Here's how the part is built. I have some questions about the finished solid (model axes, mm). Round coordinates to 2 decimals unless told otherwise and drop trailing zeros. Loops run counter-clockwise (first coordinate to the right, second up) from the corner with the lowest first, then second, coordinate; pieces in that order, holes last. Notation, with made-up numbers: M -7.75,20 L 13.25,20 A16 cw 13.25,48 Z; hole C -13.5,54 d8. An arc over 180 degrees is marked long. One line per question, with ' | ' between items. Start each with the question number.
```python
from build123d import *

# Parameters (mm, degrees)
SKETCH1_R           = 31
BOSS_EXTRUDE1_DEPTH = 2
SKETCH2_R           = 6
CUT_EXTRUDE1_DEPTH  = 2
SKETCH3_W           = 16
SKETCH3_H           = 62
BOSS_EXTRUDE2_DEPTH = 2
CUT_EXTRUDE2_REACH  = 71.347
SKETCH11_R          = 1


with BuildPart() as part:
    # Sketch1 → Boss-Extrude1 (new body)
    with BuildSketch(Plane(origin=(0, 0, 0), x_dir=(1, 0, 0), z_dir=(0, 1, 0))):
        with Locations(Location((0, 0, 0), (0, 0, 270))):
            Circle(SKETCH1_R)
    extrude(amount=BOSS_EXTRUDE1_DEPTH)

    # Sketch2 → Cut-Extrude1 (cut)
    with BuildSketch(Plane(origin=(0, 2, 0), x_dir=(1, 0, 0), z_dir=(0, 1, 0))):
        with Locations(Location((0, 0, 0), (0, 0, 270))):
            Circle(SKETCH2_R)
    extrude(amount=-CUT_EXTRUDE1_DEPTH, mode=Mode.SUBTRACT)

    # Sketch3 → Boss-Extrude2 (add)
    with BuildSketch(Plane(origin=(0, 2, 0), x_dir=(1, 0, 0), z_dir=(0, 1, 0))):
        with Locations((-23, 31)):
            Rectangle(SKETCH3_W, SKETCH3_H)
    extrude(amount=-BOSS_EXTRUDE2_DEPTH)

    # Sketch11 → Cut-Extrude2 (cut, up to next)
    with BuildSketch(Plane(origin=(0, 2, 0), x_dir=(1, 0, 0), z_dir=(0, 1, 0)), mode=Mode.PRIVATE) as cut_extrude2_sk1:
        with Locations(Location((-22.95, 54.78, 0), (0, 0, 270))):
            Circle(SKETCH11_R)
    cut_extrude2_tool1 = extrude(cut_extrude2_sk1.sketch, amount=-CUT_EXTRUDE2_REACH, mode=Mode.PRIVATE) & part.part
    add(cut_extrude2_tool1.solids().sort_by_distance((-22.95, 2, -54.78))[0], mode=Mode.SUBTRACT)


solid = part.part
```
1) Imagine slicing it at A-A (z = -54.78). Write out the boundary of the cut face in (x, y), then the cut area to 3 significant figures.
2) Imagine slicing it at C-C (x = 22.5). Write out the boundary of the cut face in (y, z), then the cut area to 3 significant figures.
3) Please list where these lines run through material, in increasing order: L1, parallel to X at y = 1.3, z = 0; L2, parallel to X at y = 0.5, z = -54.78; L3, parallel to X at y = 0.8, z = -51.5. Write a range as from..to.
4) We'd pull the mould along Z, two halves only. Please class faces 1 (the face through (-7, 0, -6)), 2 (the face through (26.11, 0.99, 16.71)), 3 (the face through (-23.56, 1.01, -55.57)): pulls with the +Z half, pulls with the -Z half, needs draft (parallel to the pull), parting line crosses it, or undercut.
5) Imagine slicing it at D-D (z = -34.5). Write out the boundary of the cut face in (x, y), then the cut area to 3 significant figures.
6) I'm going to push a flat-ended pin straight in: pin 1 Ø0.6 at (y, z) = (1, -42) entering from +X. Where does the tip first touch, or does it pass through?
7) Imagine slicing it at B-B (y = 1.5). Write out the boundary of the cut face in (x, z), then the cut area to 3 significant figures.
Results are:
1) outline: M -31,0 L -23.95,0 L -23.95,2 L -31,2 Z; M -21.95,0 L -15,0 L -15,2 L -21.95,2 Z | area: 28.0 mm²
2) outline: M 0,-21.32 L 2,-21.32 L 2,21.32 L 0,21.32 Z | area: 85.3 mm²
3) L1: -31..-6, 6..31 | L2: -31..-23.95, -21.95..-15 | L3: -31..-15
4) face 1: needs draft | face 2: parting line crosses it | face 3: undercut
5) outline: M -31,0 L -15,0 L -15,2 L -31,2 Z | area: 32.0 mm²
6) pin 1: x = -15
7) outline: M -31,-62 L -15,-62 L -15,-27.13 A31 ccw long -31,0 Z; hole C -22.95,-54.78 d2; hole C 0,0 d12 | area: 3,590 mm²
